The listing builds one solid part. Answer for the finished solid, in the listing's coordinates (mm). Face numbers are marked on the shaded views. A direction names the side the tool comes from. Give positions to 0.01 mm unless a question says otherwise; leave off trailing zeros. Write each loop counter-clockwise with the first axis right and the second up, starting at its lowest first coordinate (ties: lowest second). Pieces come first, ordered by that corner, then holes. Notation, with made-up numbers: M 15,-11 L 59,-11 A34 cw 59,27 Z; hole C -17,3.5 d2. An arc over 180 degrees is marked long. Answer as a JSON object with one key per item and string values.
```python
from build123d import *

# Parameters (mm, degrees)
F0_R     = 50
F1_DEPTH = 20
F2_W     = 12
F2_H     = 130.80296
F3_DEPTH = 10
F4_R     = 30
F5_DEPTH = 30
F7_W     = 3
F7_H     = 6
F8_DEPTH = 10
F6_R     = 15
F9_DEPTH = 50.001


with BuildPart() as f1:
    # F0 (on Top) → F1 (new body)
    with BuildSketch(Plane.XY):
        Circle(F0_R)
    extrude(amount=F1_DEPTH)

    # F2 (on face) → F3 (cut)
    with BuildSketch(Plane.XY.offset(20)):
        Rectangle(F2_W, F2_H)
    extrude(amount=-F3_DEPTH, mode=Mode.SUBTRACT)

    # F4 (on face) → F5 (join)
    with BuildSketch(Plane(origin=(0, 0, 0), x_dir=(1, 0, 0), z_dir=(0, 0, -1))):
        Circle(F4_R)
    extrude(amount=F5_DEPTH)

    # F7 (on face) → F8 (cut)
    with BuildSketch(Plane(origin=(0, 0, -30), x_dir=(1, 0, 0), z_dir=(0, 0, -1))):
        with Locations((15, 0)):
            Rectangle(F7_W, F7_H)
    extrude(amount=-F8_DEPTH, mode=Mode.SUBTRACT)

    # F6 (on face) → F9 (cut, through all)
    with BuildSketch(Plane(origin=(0, 0, -30), x_dir=(1, 0, 0), z_dir=(0, 0, -1))):
        Circle(F6_R)
    extrude(amount=-F9_DEPTH, mode=Mode.SUBTRACT)


solid = f1.part
```
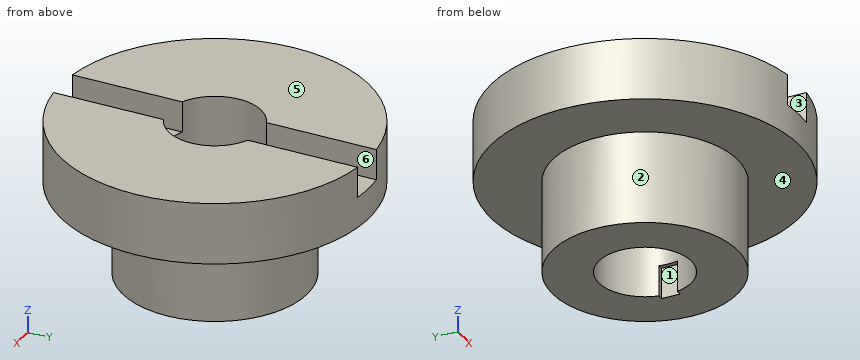
1. For the marked faces 4, 5 and 6, determine the directions among +Z, -Z, +X, -X, +Y, -Y from which every point of the face is accessible in a straight line to the end or side of a thin tool.
Verdict:
{"face 4": "-Z", "face 5": "+Z, +X, -X, +Y, -Y", "face 6": "+Z, +Y, -Y"}
2. Flat-ended cylindrical pins translate along their axes: pin 1 (2 mm diameter, centred on y = 27.5, z = 13.5, fed in from +X); pin 2 (5 mm diameter, centred on y = -25, z = 14.5, fed in from +X); pin 3 (6.5 mm diameter, centred on y = -1, z = -27, fed in from -X); pin 4 (18 mm diameter, centred on x = 0, y = 0, fed in from +Z). Find the tip coordinate at first contact, or state that the pin passes through.
Verdict:
{"pin 1": "stops at x = 42.4", "pin 2": "stops at x = 44.65", "pin 3": "stops at x = -30", "pin 4": "passes through"}
3. A cutting plane is placed at D-D, the plane z = -18.5. Give the vertices of the cut face in (x, y).
Verdict:
{"outline": "C 0,0 d60; hole C 0,0 d30"}
4. A cutting plane is placed at B-B, the plane x = 0. Give the vertices of the cut face in (y, z), plus the area to 3 significant figures.
Verdict:
{"outline": "M -50,0 L -30,0 L -30,-30 L -15,-30 L -15,10 L -50,10 Z; M 15,-30 L 30,-30 L 30,0 L 50,0 L 50,10 L 15,10 Z", "area": "1,600 mm2"}
5. A cutting plane is placed at A-A, the plane z = 15.5. Give the vertices of the cut face in (x, y), plus the area to 3 significant figures.
Verdict:
{"outline": "M -6,-49.64 L -6,-13.75 A15 cw -6,13.75 L -6,49.64 A50 ccw Z; M 6,-49.64 A50 ccw 6,49.64 L 6,13.75 A15 cw 6,-13.75 Z", "area": "6,300 mm2"}
6. Consider line 1 along X through (y, z) = (0, 1); line 2 along X through (y, z) = (0, -7.5). Determine where each line is inside the solid, lowest interval first.
Verdict:
{"line 1": "x = -50 to -15, 15 to 50", "line 2": "x = -30 to -15, 15 to 30"}
7. A cutting plane is placed at C-C, the plane y = 0. Give the vertices of the cut face in (x, z).
Verdict:
{"outline": "M -50,0 L -30,0 L -30,-30 L -15,-30 L -15,20 L -50,20 Z; M 15,-20 L 16.5,-20 L 16.5,-30 L 30,-30 L 30,0 L 50,0 L 50,20 L 15,20 Z"}
8. The mould has two halves that part along Y. Classify the marked faces 1, 2 and 3: released by +Y, released by -Y, zero draft, split by the parting line, or undercut.
Verdict:
{"face 1": "undercut", "face 2": "split by the parting line", "face 3": "zero draft"}
